```python
from build123d import *

# Parameters (mm, degrees)
F1_DEPTH = 50.8
F2_R     = 23.0676038816
F3_DEPTH = 130.048
F4_W     = 88.9319777489
F4_H     = 51.5172313899
F5_DEPTH = 12.7
F7_DEPTH = 3.175


with BuildPart() as f1:
    # F0 (on Top) → F1 (new body)
    with BuildSketch(Plane.XY):
        with BuildLine():
            ThreePointArc((16.3361351828, -31.75), (57.1135301245, -34.8840355997), (78.4611805258, 0))
            ThreePointArc((78.4611805258, 0), (57.1135301245, 34.8840355997), (16.3361351828, 31.75))
            Line((16.3361351828, 31.75), (29.5000914484, 31.75))
            Line((29.5000914484, 31.75), (29.5000914484, -31.75))
            Line((29.5000914484, -31.75), (16.3361351828, -31.75))
        make_face()
        with BuildLine():
            Line((29.5000914484, 31.75), (16.3361351828, 31.75))
            ThreePointArc((16.3361351828, 31.75), (0.109788877, 0), (16.3361351828, -31.75))
            Line((16.3361351828, -31.75), (29.5000914484, -31.75))
            Line((29.5000914484, -31.75), (29.5000914484, 31.75))
        make_face()
    extrude(amount=F1_DEPTH)

    # F2 (on Top) → F3 (cut)
    with BuildSketch(Plane.XY):
        with Locations((37.608332932, 0)):
            Circle(F2_R)
    extrude(amount=F3_DEPTH, mode=Mode.SUBTRACT)

    # F4 (on Top) → F5 (join)
    with BuildSketch(Plane.XY):
        with Locations((-31.6792652011, 0.5756122991)):
            Rectangle(F4_W, F4_H)
    extrude(amount=F5_DEPTH)

    # F6 (on Front) → F7 (join, symmetric)
    with BuildSketch(Plane.XZ):
        Polygon((0, 0), (0, 33.8171757758), (-66.6476637125, 0), align=None)
    extrude(amount=F7_DEPTH, both=True)


solid = f1.part
```
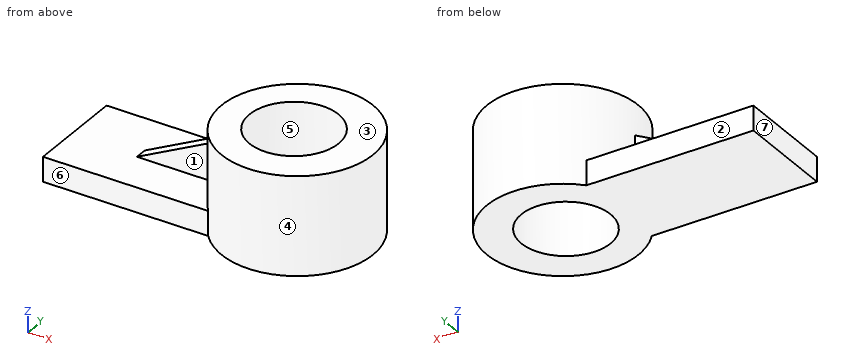
The model under review builds one solid part; all positions refer to its coordinate system, in mm. Face numbers are marked on the shaded views. A direction names the side the tool comes from. Round coordinates to 2 decimals unless told otherwise and drop trailing zeros. Loops run counter-clockwise (first coordinate to the right, second up) from the corner with the lowest first, then second, coordinate; pieces in that order, holes last.
1) Wall thickness on line 1 along X through (y, z) = (0.5, 42); line 2 along Z through (x, y) = (-4, 17); line 3 along X through (y, z) = (-1, 6): over which ranges is each line inside the solid? List them lowest first.
Values follow:
line 1: x = 0.11 to 14.55, 60.67 to 78.46
line 2: z = 0 to 12.7
line 3: x = -76.15 to 14.56, 60.65 to 78.45
2) Tool access review of the marked faces 1, 2, 3 and 4: name each direction out of +Z, -Z, +X, -X, +Y, -Y from which nothing blocks a thin tool from reaching the whole face with its end or side.
Values follow:
face 1: +Z, -X, -Y
face 2: +Z, -Z, -X, +Y
face 3: +Z, +X, -X, +Y, -Y
face 4: +Z
3) Clearance check with flat-ended pins moving along their axes: P1, Ø17, axis at x = -18.5, z = 25.5, coming from the -Y side (3 decimals); P2, Ø4, axis at x = -45, z = 9.5, coming from the +Y side; P3, Ø8, axis at x = -1.5, y = 22, coming from the +Z side. State where each tip first meets the part, or that it passes through.
Values follow:
P1: stops at y = -3.175
P2: stops at y = 26.33
P3: stops at z = 12.7
4) Consider section D-D on z = 30.5. State the section outline as (x, y) points (3 decimals).
Values follow:
outline: (-6.538, -3.175) - (0, -3.175) - (0, 3.175) - (-6.538, 3.175) - close; circle Ø78.351 at (39.285, 0); hole circle Ø46.135 at (37.608, 0)
5) Consider section A-A on y = 0. State the section outline as (x, z) points, then the cut area to 3 significant figures.
Values follow:
outline: (-76.15, 0) - (14.54, 0) - (14.54, 50.8) - (0.11, 50.8) - (0.11, 12.7) - (0, 12.7) - (0, 33.82) - (-41.62, 12.7) - (-76.15, 12.7) - close; (60.68, 0) - (78.46, 0) - (78.46, 50.8) - (60.68, 50.8) - close
area: 3,040 mm2
6) The part is to be moulded in two halves that separate along X. For the marked faces 5, 6 and 7, say which applies: pulls with the +X half, pulls with the -X half, needs draft (parallel to the pull), parting line crosses it, or undercut.
Values follow:
face 5: undercut
face 6: needs draft
face 7: pulls with the -X half
7) Consider section C-C on x = 43. State the section outline as (y, z) points.
Values follow:
outline: (-39, 0) - (-22.43, 0) - (-22.43, 50.8) - (-39, 50.8) - close; (22.43, 0) - (39, 0) - (39, 50.8) - (22.43, 50.8) - close
8) Consider section B-B on z = 10.5. State the section outline as (x, y) points.
Values follow:
outline: (-76.15, -25.18) - (9.28, -25.18) arc R39.18 ccw (long way) to (10.28, 26.33) - (-76.15, 26.33) - close; hole circle Ø46.14 at (37.61, 0)
